Can you work these out from the model? Positions are in its coordinate system, mm. Face numbers are marked on the shaded views. A direction names the side the tool comes from. Coordinates: 2 decimals unless noted, no trailing zeros. Loops run counter-clockwise (first coordinate to the right, second up) from the corner with the lowest first, then second, coordinate; pieces in that order, holes last.
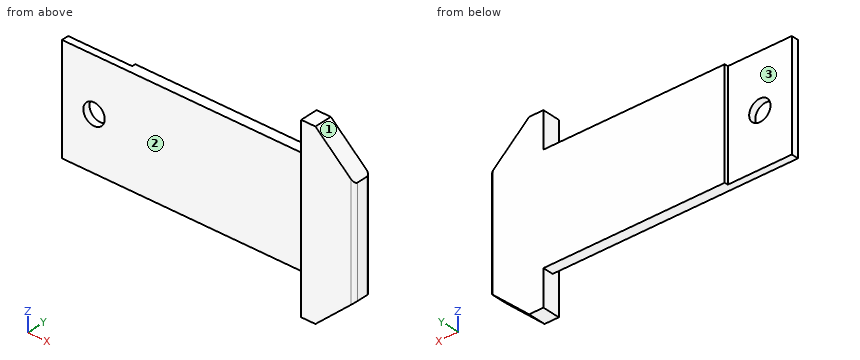
```python
from build123d import *

# Parameters (mm, degrees)
F0_W     = 42
F0_H     = 15
F1_DEPTH = 1.5
F2_R     = 1.5
F3_DEPTH = 1.501
F5_DEPTH = 1.5
F6_W     = 9
F6_H     = 0.5
F7_DEPTH = 20.001
F9_DEPTH = 1
F10_R    = 0.5


with BuildPart() as f1:
    # F0 (on Front) → F1 (new body)
    with BuildSketch(Plane.XZ):
        with Locations((4, 0)):
            Rectangle(F0_W, F0_H)
    extrude(amount=F1_DEPTH)

    # F2 (on face) → F3 (cut, through all)
    with BuildSketch(Plane.XZ.offset(1.5)):
        with Locations((-12.5, 0)):
            Circle(F2_R)
    extrude(amount=-F3_DEPTH, mode=Mode.SUBTRACT)

    # F4 (on face) → F5 (join, through all)
    with BuildSketch(Plane.XZ.offset(1.5)):
        Polygon((19.5, -12.5), (25, -7.5), (17.5, -7.5), (17.5, -12.5), align=None)
        Polygon((17.5, 7.5), (25, 7.5), (19.5, 12.5), (17.5, 12.5), align=None)
    extrude(amount=-F5_DEPTH)

    # F6 (on face) → F7 (cut, through all)
    with BuildSketch(Plane(origin=(0, 0, -7.5), x_dir=(1, 0, 0), z_dir=(0, 0, -1))):
        with Locations((-12.5, 0.25)):
            Rectangle(F6_W, F6_H)
    extrude(amount=-F7_DEPTH, mode=Mode.SUBTRACT)

    # F8 (on face) → F9 (join)
    with BuildSketch(Plane.XZ.offset(1.5)):
        Polygon((25, 7.5), (19.5, 12.5), (17.5, 12.5), (17.5, -12.5), (19.5, -12.5), (25, -7.5), align=None)
    extrude(amount=F9_DEPTH)

    # F10
    f10_edges = [f1.edges().sort_by_distance(p)[0] for p in [
        (25, -2.5, 0),
        (25, 0, 0),
    ]]
    fillet(f10_edges, radius=F10_R)


solid = f1.part
```
Item 1: Suppose I cut it at C-C, the plane x = -12.5. Please give me the cut outline in (y, z).
Results are:
outline: (-1.5, -7.5) - (-0.5, -7.5) - (-0.5, -1.5) - (-1.5, -1.5) - close; (-1.5, 1.5) - (-0.5, 1.5) - (-0.5, 7.5) - (-1.5, 7.5) - close
Item 2: Suppose I cut it at D-D, the plane z = -4.75. Please give me the cut outline in (x, y), plus the area to 3 significant figures.
Results are:
outline: (-17, -1.5) - (17.5, -1.5) - (17.5, -2.5) - (24.5, -2.5) arc R0.5 ccw to (25, -2) - (25, -0.5) arc R0.5 ccw to (24.5, 0) - (-8, 0) - (-8, -0.5) - (-17, -0.5) - close
area: 65.9 mm2
Item 3: Suppose I cut it at B-B, the plane y = -0.95. Please give me the cut outline in (x, z).
Results are:
outline: (-17, -7.5) - (17.5, -7.5) - (17.5, -12.5) - (19.5, -12.5) - (25, -7.5) - (25, 7.5) - (19.5, 12.5) - (17.5, 12.5) - (17.5, 7.5) - (-17, 7.5) - close; hole circle Ø3 at (-12.5, 0)
Item 4: I'm going to push flat-ended pins straight in: P1, Ø4, axis at x = -12.5, z = 0, coming from the +Y side; P2, Ø0.8, axis at x = 9, y = -0.5, coming from the -Z side; P3, Ø0.6, axis at y = 0, z = 0.5, coming from the -X side. Where does each tip first touch, or does it pass through?
Results are:
P1: stops at y = -0.5
P2: stops at z = -7.5
P3: stops at x = -8
Item 5: Suppose I cut it at A-A, the plane z = 0. Please give me the cut outline in (x, y).
Results are:
outline: (-17, -1.5) - (-14, -1.5) - (-14, -0.5) - (-17, -0.5) - close; (-11, -1.5) - (17.5, -1.5) - (17.5, -2.5) - (24.5, -2.5) arc R0.5 ccw to (25, -2) - (25, -0.5) arc R0.5 ccw to (24.5, 0) - (-8, 0) - (-8, -0.5) - (-11, -0.5) - close
Item 6: I need wall thicknesses on line 1 along Z through (x, y) = (-12.5, -0.95); line 2 along Z through (x, y) = (16.5, -0.75); line 3 along Y through (x, z) = (-5.5, -3.25). Which ranges of each line are inside material? Lowest first, please.
Results are:
line 1: z = -7.5 to -1.5, 1.5 to 7.5
line 2: z = -7.5 to 7.5
line 3: y = -1.5 to 0
Item 7: On a 3-axis mill with a long thin cutter (end or side, diameter ignored), from which of +Z, -Z, +X, -X, +Y, -Y can I reach the whole of each face in a straight line? I mean the marked faces 1, 2 and 3. Say none if no direction works.
Results are:
face 1: +Z, +X, +Y, -Y
face 2: +Z, -Z, -X, -Y
face 3: +Z, -Z, -X, +Y
